Read the model definition and answer for the solid it produces. Units are mm, in the model's axes. Face numbers are marked on the shaded views. A direction names the side the tool comes from. Coordinates: 2 decimals unless noted, no trailing zeros. Write each loop counter-clockwise with the first axis right and the second up, starting at its lowest first coordinate (ties: lowest second). Pieces come first, ordered by that corner, then holes. Notation, with made-up numbers: (72.5, -5.75) -> (111.5, -5.75) arc R16 cw to (111.5, 12.25) -> close; hole circle Ø9 at (59.5, 31.5). An arc over 180 degrees is marked (long way). Answer as a JSON object with one key per item and string values. Group by question number.
(1) Find section D-D (y = -10.5). Give the vertices of the cut face in (x, z), then the cut area to 3 significant figures.
(2) Find section A-A (x = -10). Give the vertices of the cut face in (y, z).
(3) Find section C-C (z = -45). Give the vertices of the cut face in (x, y), then the cut area to 3 significant figures.
(4) Which of the six approach directions +Z, -Z, +X, -X, +Y, -Y give full straight-line access (tool end or side, diameter ignored) to the marked faces 4 and 5?
(5) Flat-ended cylindrical pins translate along their axes: P1, Ø8, axis at x = -47.5, y = 14, coming from the +Z side; P2, Ø10, axis at x = -14.5, z = -27, coming from the -Y side; P3, Ø21, axis at x = -65.5, y = 42, coming from the +Z side. Find the tip coordinate at first contact, or state that the pin passes through.
(6) For a pull along Y with two mould halves and no side action, classify the marked faces 1, 2 and 3 as +Y half, -Y half, draft (parallel to the pull), parting line (faces both ways), or undercut.
(7) Straight lines are drawn through the part: L1, parallel to X at y = -13.5, z = -12; L2, parallel to X at y = 11, z = -53; L3, parallel to X at y = 53, z = -8. For each, find the intervals that lie inside material, in ascending order.
(8) Find section B-B (z = -20.5). Give the vertices of the cut face in (x, y), then the cut area to 3 significant figures.
from build123d import *

# Parameters (mm, degrees)
F0_W        = 198.8127231598
F0_H        = 127.7878135443
F1_DEPTH    = 100.584
F2_T1_DEPTH = 706.7873225248
F3_W        = 90.9917657264
F3_H        = 25.9568989277
F4_DEPTH    = 88.392
F5_W        = 89.8508075625
F5_H        = 26.2421388179
F6_DEPTH    = 88.646
F7_DEPTH    = 0.254
F8_DEPTH    = 0.254
F9_W        = 90.7065253705
F9_H        = 9.6981823444
F10_DEPTH   = 90.678
F11_W       = 90.4212845489
F11_H       = 39.0779660083
F11_W_2     = 33.3731551655
F11_H_2     = 51.9137959927
F11_W_3     = 52.7695268393
F12_DEPTH   = 88.646


# Not quite as in the source:
# - a fillet or chamfer that OpenCascade refuses, or shapes differently, is made with other operations: its cross-section is extruded or revolved along the edge and cut away or added


with BuildPart() as f1:
    # F0 (on Top) → F1 (new body)
    with BuildSketch(Plane.XY):
        with Locations((-0.7131025195, -5.5621936917)):
            Rectangle(F0_W, F0_H)
    extrude(amount=-F1_DEPTH)

    # F2: fillet of radius 101.6 on 1 edges, made by hand

    # F2_s2 → F2_t1 (cut)
    with BuildSketch(Plane.YZ.offset(-354.1067637819)):
        with BuildLine():
            ThreePointArc((-69.4561004639, -100.584), (-39.3431167706, -29.39963435), (32.1388194091, 0))
            Line((32.1388194091, 0), (-69.4561004639, 0))
            Line((-69.4561004639, 0), (-69.4561004639, -100.584))
        make_face()
    extrude(amount=F2_T1_DEPTH, mode=Mode.SUBTRACT)

    # F3 (on Top) → F4 (cut)
    with BuildSketch(Plane.XY):
        with Locations((-50.2023545559, 41.3598939776)):
            Rectangle(F3_W, F3_H)
    extrude(amount=-F4_DEPTH, mode=Mode.SUBTRACT)

    # F5 (on Top) → F6 (cut)
    with BuildSketch(Plane.XY):
        with Locations((49.631874077, 41.2172740325)):
            Rectangle(F5_W, F5_H)
    extrude(amount=-F6_DEPTH, mode=Mode.SUBTRACT)

    # F7 (cut): a face of the model
    f7_faces = [f1.faces().sort_by_distance(p)[0] for p in [
        (-50.2023545559, 41.3598939776, -88.392),
    ]]
    extrude(f7_faces, amount=F7_DEPTH, mode=Mode.SUBTRACT)

    # F8 (cut): a face of the model
    f8_faces = [f1.faces().sort_by_distance(p)[0] for p in [
        (49.631874077, 41.2172740325, -88.646),
    ]]
    extrude(f8_faces, amount=-F8_DEPTH, mode=Mode.SUBTRACT)

    # F9 (on Top) → F10 (cut)
    with BuildSketch(Plane.XY):
        with Locations((-50.3449747339, 13.5489311069)):
            Rectangle(F9_W, F9_H)
    extrude(amount=-F10_DEPTH, mode=Mode.SUBTRACT)

    # F11 (on Top) → F12 (cut)
    with BuildSketch(Plane.XY):
        with Locations((-50.4875951447, -13.9767907094)):
            Rectangle(F11_W, F11_H)
        with Locations((21.1078075226, -7.5588757172)):
            Rectangle(F11_W_2, F11_H_2)
        with Locations((67.8872764111, -7.5588757172)):
            Rectangle(F11_W_3, F11_H_2)
    extrude(amount=-F12_DEPTH, mode=Mode.SUBTRACT)


solid = f1.part
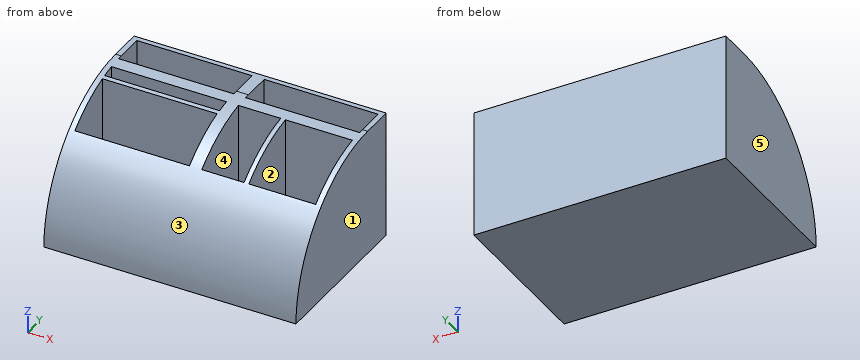
Results below:
{
 "1": {"outline": "(-100.12, -100.58) -> (98.69, -100.58) -> (98.69, -9.38) -> (94.27, -9.38) -> (94.27, -88.65) -> (41.5, -88.65) -> (41.5, -9.38) -> (37.79, -9.38) -> (37.79, -88.65) -> (4.42, -88.65) -> (4.42, -9.38) -> (-5.28, -9.38) -> (-5.28, -88.65) -> (-95.7, -88.65) -> (-95.7, -9.38) -> (-100.12, -9.38) -> close", "area": "4,140 mm2"},
 "2": {"outline": "(-69.46, -100.58) -> (58.33, -100.58) -> (58.33, 0) -> (54.34, 0) -> (54.34, -88.39) -> (28.38, -88.39) -> (28.38, -0.07) arc R101.6 ccw to (18.4, -0.93) -> (18.4, -90.68) -> (8.7, -90.68) -> (8.7, -2.74) arc R101.6 ccw to (5.56, -3.54) -> (5.56, -88.65) -> (-33.52, -88.65) -> (-33.52, -24.06) arc R101.6 ccw to start"},
 "3": {"outline": "(-100.12, -52.24) -> (98.69, -52.24) -> (98.69, 58.33) -> (-100.12, 58.33) -> close; hole (-95.7, -33.52) -> (-5.28, -33.52) -> (-5.28, 5.56) -> (-95.7, 5.56) -> close; hole (-95.7, 8.7) -> (-4.99, 8.7) -> (-4.99, 18.4) -> (-95.7, 18.4) -> close; hole (-95.7, 28.38) -> (-4.71, 28.38) -> (-4.71, 54.34) -> (-95.7, 54.34) -> close; hole (4.42, -33.52) -> (37.79, -33.52) -> (37.79, 18.4) -> (4.42, 18.4) -> close; hole (4.71, 28.1) -> (94.56, 28.1) -> (94.56, 54.34) -> (4.71, 54.34) -> close; hole (41.5, -33.52) -> (94.27, -33.52) -> (94.27, 18.4) -> (41.5, 18.4) -> close", "area": "8,380 mm2"},
 "4": {"face 4": "+Z", "face 5": "+Z, -Z, -X, +Y, -Y"},
 "5": {"P1": "stops at z = -90.68", "P2": "stops at y = -41.88", "P3": "stops at z = -88.39"},
 "6": {"face 1": "draft", "face 2": "undercut", "face 3": "-Y half"},
 "7": {"L1": "x = -100.12 to -95.7, -5.28 to 4.42, 37.79 to 41.5, 94.27 to 98.69", "L2": "x = -100.12 to -95.7, -4.99 to 4.42, 37.79 to 41.5, 94.27 to 98.69", "L3": "x = -100.12 to -95.7, -4.71 to 4.71, 94.56 to 98.69"},
 "8": {"outline": "(-100.12, -29.06) -> (-95.7, -29.06) -> (-95.7, 5.56) -> (-5.28, 5.56) -> (-5.28, -29.06) -> (4.42, -29.06) -> (4.42, 18.4) -> (37.79, 18.4) -> (37.79, -29.06) -> (41.5, -29.06) -> (41.5, 18.4) -> (94.27, 18.4) -> (94.27, -29.06) -> (98.69, -29.06) -> (98.69, 58.33) -> (-100.12, 58.33) -> close; hole (-95.7, 8.7) -> (-4.99, 8.7) -> (-4.99, 18.4) -> (-95.7, 18.4) -> close; hole (-95.7, 28.38) -> (-4.71, 28.38) -> (-4.71, 54.34) -> (-95.7, 54.34) -> close; hole (4.71, 28.1) -> (94.56, 28.1) -> (94.56, 54.34) -> (4.71, 54.34) -> close", "area": "4,560 mm2"}
}
